Can you work these out from the model? Positions are in its coordinate system, mm. Face numbers are marked on the shaded views. A direction names the side the tool comes from. Give positions to 0.01 mm unless a question says otherwise; leave off trailing zeros. Write each loop counter-clockwise with the first axis right and the second up, starting at its lowest first coordinate (ties: lowest second). Pieces come first, ordered by that corner, then holes.
```python
from build123d import *
from build123d.topology import SkipClean

# Parameters (mm, degrees)
BOSS_EXTRUDE1_DEPTH     = 7
CUT_EXTRUDE1_DEPTH      = 78.980769199
CUT_EXTRUDE1_DEPTH_BACK = 78.980769199
SKETCH3_R               = 2.75
SKETCH4_R               = 12.1
CUT_EXTRUDE2_DEPTH      = 5.1
BOSS_EXTRUDE2_START     = 0.5
SKETCH5_R               = 4.25
SKETCH5_R_2             = 2.75
BOSS_EXTRUDE2_DEPTH     = 0.5
SKETCH6_R               = 5.1
CUT_EXTRUDE3_DEPTH      = 3.5
FILLET1_R               = 5
CUT_EXTRUDE4_DEPTH      = 3.5


with BuildPart() as part:
    # Sketch1 → Boss-Extrude1 (new body)
    with BuildSketch(Plane.XY):
        with BuildLine():
            Line((64.000002369, 34.999998632), (64.000002369, 7.0000007))
            ThreePointArc((64.000002369, 7.0000007), (59.061035156, 0.310296383), (51.213675554, 3.060657863))
            Line((51.213675554, 3.060657863), (47.766721553, 8.123736451))
            ThreePointArc((47.766721553, 8.123736451), (43.713065604, 11.089441566), (38.696960231, 10.832108598))
            ThreePointArc((38.696960231, 10.832108598), (35.414081121, 9.836258221), (32.00000085, 9.5000007))
            Line((32.00000085, 9.5000007), (32.00000085, 15.4000007))
            ThreePointArc((32.00000085, 15.4000007), (43.60000085, 27.0000007), (32.00000085, 38.6000007))
            Line((32.00000085, 38.6000007), (32.00000085, 44.0000007))
            ThreePointArc((32.00000085, 44.0000007), (36.123106475, 43.492423203), (40.00000085, 42.0000007))
            Line((40.00000085, 42.0000007), (57.000002369, 42.0000007))
            ThreePointArc((57.000002369, 42.0000007), (61.9497513, 39.949747563), (64.000002369, 34.999998632))
        make_face()
    extrude(amount=BOSS_EXTRUDE1_DEPTH)

    # Sketch3 → Cut-Extrude1 (cut, two sides: drawn at the far end of the back side and taken through both)
    with BuildSketch(Plane.XY.offset(7).offset(-CUT_EXTRUDE1_DEPTH_BACK)):
        with Locations((56.999999697, 35.000001537)):
            Circle(SKETCH3_R)
        with Locations((56.999999697, 19.000001537)):
            Circle(SKETCH3_R)
        with Locations((56.999999697, 7.000001537)):
            Circle(SKETCH3_R)
    extrude(amount=CUT_EXTRUDE1_DEPTH + CUT_EXTRUDE1_DEPTH_BACK, mode=Mode.SUBTRACT)

    # Sketch4 → Cut-Extrude2 (cut)
    with BuildSketch(Plane(origin=(0, 0, 0), x_dir=(-1, 0, 0), z_dir=(0, 0, -1))):
        with Locations((-32.00000085, 27.0000007)):
            Circle(SKETCH4_R)
    extrude(amount=-CUT_EXTRUDE2_DEPTH, mode=Mode.SUBTRACT)

    # Sketch5 → Boss-Extrude2 (add)
    with BuildSketch(Plane.XY.offset(7).offset(BOSS_EXTRUDE2_START)):
        with Locations((56.999999697, 7.000001537)):
            Circle(SKETCH5_R)
        with Locations((56.999999697, 7.000001537)):
            Circle(SKETCH5_R_2, mode=Mode.SUBTRACT)
    extrude(amount=-BOSS_EXTRUDE2_DEPTH)

    # Sketch6 → Cut-Extrude3 (cut)
    with BuildSketch(Plane.XY.offset(7)):
        with Locations((56.999999697, 19.000001537)):
            Circle(SKETCH6_R)
        with Locations((56.999999697, 35.000001537)):
            Circle(SKETCH6_R)
    extrude(amount=-CUT_EXTRUDE3_DEPTH, mode=Mode.SUBTRACT)

    # Fillet1
    fillet1_edges = [part.edges().sort_by_distance(p)[0] for p in [
        (40.00000085, 42.0000007, 3.5),
    ]]
    fillet(fillet1_edges, radius=FILLET1_R)

    # Sketch8 → Cut-Extrude4 (cut)
    with BuildSketch(Plane(origin=(0, 0, 0), x_dir=(-1, 0, 0), z_dir=(0, 0, -1))):
        Polygon((-54.546261053, 11.250001537), (-59.453738341, 11.250001537), (-61.907476985, 7.000001537), (-59.453738341, 2.750001537), (-54.546261053, 2.750001537), (-52.092522409, 7.000001537), align=None)
    extrude(amount=-CUT_EXTRUDE4_DEPTH, mode=Mode.SUBTRACT)

    # Mirror2: part across plane


with BuildPart() as part_1:
    with SkipClean():  # the faces are left unmerged after this step: merging them gives an invalid solid
        add(part.part)
        add(part.part.mirror(Plane(origin=(32.00000085, 44.0000007, 7), x_dir=(0, 0, 1), z_dir=(1, 0, 0))))


solid = part_1.part
```
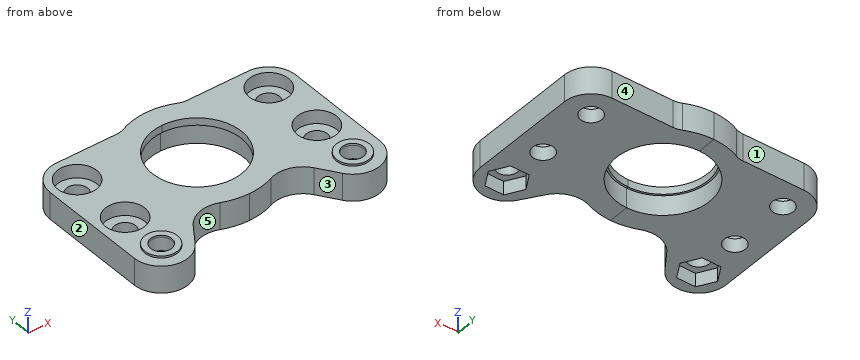
1) For the marked faces 4 and 5, which set-ups out of +Z, -Z, +X, -X, +Y, -Y let a thin tool reach every point of the face, with its end or its side?
Values follow:
face 4: +Z, -Z, +X, +Y
face 5: +Z, -Z, -Y
2) Suppose I cut it at D-D on x = 10.5. Write out the boundary of the cut face in (y, z).
Values follow:
outline: (0.94, 0) - (4.56, 0) - (4.56, 3.5) - (9.44, 3.5) - (9.44, 0) - (42, 0) - (42, 7) - (38.71, 7) - (38.71, 3.5) - (31.29, 3.5) - (31.29, 7) - (22.71, 7) - (22.71, 3.5) - (15.29, 3.5) - (15.29, 7) - (9.41, 7) - (9.41, 7.5) - (4.59, 7.5) - (4.59, 7) - (0.94, 7) - close
3) Suppose I cut it at C-C on z = 1. State how many separate pieces and enclosed holes the cut face has, plus the area to 3 significant figures.
Values follow:
separate pieces: 1
enclosed holes: 7
area: 1,610 mm2
4) For pin 1 Ø1 at (x, z) = (10, 5.5) entering from +Y; pin 2 Ø11 at (x, y) = (6.5, 17.5) entering from +Z; pin 3 Ø2 at (x, z) = (25.5, 1.5) entering from -Y, each with a flat end and sliding along its axis, tell me the tip position at first contact or that it passes through.
Values follow:
pin 1: stops at y = 42
pin 2: stops at z = 7
pin 3: stops at y = 10.39
5) If we mould it in two halves opening along X, with no side actions, what happens to the marked faces 1, 2 and 3? For each: +X half, -X half, draft (parallel to the pull), parting line (faces both ways), or undercut.
Values follow:
face 1: draft
face 2: -X half
face 3: undercut
6) Suppose I cut it at A-A on y = 27. Write out the boundary of the cut face in (x, z), plus the area to 4 significant figures.
Values follow:
outline: (0, 0) - (19.9, 0) - (19.9, 5.1) - (20.4, 5.1) - (20.4, 7) - (0, 7) - close; (43.6, 5.1) - (44.1, 5.1) - (44.1, 0) - (64, 0) - (64, 7) - (43.6, 7) - close
area: 280.5 mm2
7) Suppose I cut it at B-B on x = 29.5. Write out the boundary of the cut face in (y, z).
Values follow:
outline: (9.68, 0) - (15.16, 0) - (15.16, 5.1) - (15.67, 5.1) - (15.67, 7) - (9.68, 7) - close; (38.33, 5.1) - (38.84, 5.1) - (38.84, 0) - (43.82, 0) - (43.82, 7) - (38.33, 7) - close
8) Please list where these lines run through material, in increasing order: L1, parallel to Y at x = 9, z = 4.5; L2, parallel to X at y = 34.5, z = 5.5; L3, parallel to Y at x = 6.5, z = 4.25.
Values follow:
L1: y = 0.29 to 5.11, 8.89 to 14.31, 23.69 to 30.31, 39.69 to 42
L2: x = 0 to 1.92, 12.08 to 23.15, 40.85 to 51.92, 62.08 to 64
L3: y = 0.02 to 4.3, 9.7 to 13.92, 24.08 to 29.92, 40.08 to 41.98
